Geometry check sheet. Reference: the model listing, model coordinates, mm. A direction names the side the tool comes from. Give positions to 0.01 mm unless a question says otherwise; leave off trailing zeros. Write each loop counter-clockwise with the first axis right and the second up, starting at its lowest first coordinate (ties: lowest second). Pieces come first, ordered by that corner, then holes. Notation, with made-up numbers: (56, 20) - (60, 20) arc R20 ccw to (60, 55) - close; hole circle Ø5 at (64, 39.5). An arc over 180 degrees is marked (long way). One line per question, with ' | ' between items. Start each with the question number.
Q1. Release check for a two-part mould opening along X. For faces 5 (the face through (-2.1, -12.4, 0)), 6 (the face through (0, -7, -14)), 7 (the face through (-8.767, -16.856, 2.902)) record: +X half, -X half, draft (parallel to the pull), parting line (faces both ways), or undercut.
Q2. Section check C-C on z = -1.25. Record the boundary of the cut face in (x, y).
Q3. Thickness scan on L1, parallel to Y at x = 0, z = -11.65; L2, parallel to X at y = -11, z = 6.5; L3, parallel to Y at x = -11, z = -0.75. Record the ranges inside material, lowest first. Write a range as [from, to].
Q4. Set-up check for faces 1 (the face through (-5.72, -11, 0.74)), 2 (the face through (-10.7, 10.4, 2.9)), 3 (the face through (1.5, 9, -13.5)), 4 (the face through (-5.602, 0.9, -13.5)): record each of +Z, -Z, +X, -X, +Y, -Y from which the full face is reachable in a straight line by a thin tool's end or side.
Q5. Gauge pin test, flat ends, axial feed: P1, Ø8.5, axis at x = 5, y = 4.5, coming from the +Z side; P2, Ø1, axis at x = 7, z = -2.5, coming from the +Y side; P3, Ø1.1, axis at y = 1.5, z = -13.5, coming from the -X side. Record the tip position at first contact, or that the pin passes through.
Q6. Section check D-D on x = 15. Record the boundary of the cut face in (y, z).
```python
from build123d import *

# Parameters (mm, degrees)
F2_R     = 1.1
F3_DEPTH = 14
F5_DEPTH = 1


with BuildPart() as f1:
    # F0 (on Front) → F1 (revolve)
    with BuildSketch(Plane.XZ):
        with BuildLine():
            Line((-14, 0), (-14, 9.5))
            ThreePointArc((-14, 9.5), (-14.146447, 9.853553), (-14.5, 10))
            Line((-14.5, 10), (-19, 10))
            Line((-19, 10), (-19, -4))
            Line((-19, -4), (-11, -4))
            Line((-11, -4), (-11, -14))
            Line((-11, -14), (-4, -14))
            Line((-4, -14), (-4, -8.1))
            Line((-4, -8.1), (-9.6, -2.5))
            Line((-9.6, -2.5), (-9.6, 1.5))
            ThreePointArc((-9.6, 1.5), (-9.746447, 1.853553), (-10.1, 2))
            Line((-10.1, 2), (-11.9, 2))
            ThreePointArc((-11.9, 2), (-12.253553, 1.853553), (-12.4, 1.5))
            Line((-12.4, 1.5), (-12.4, 0))
            Line((-12.4, 0), (-14, 0))
        make_face()
    revolve(axis=Axis((0, 0, -7), (0, 0, -1)))

    # F2 (on face) → F3 (cut, through all)
    with BuildSketch(Plane(origin=(0, 0, -4), x_dir=(1, 0, 0), z_dir=(0, 0, -1))):
        with Locations((11.313708, 11.313708)):
            Circle(F2_R)
        with Locations((-11.313708, -11.313708)):
            Circle(F2_R)
        with Locations((11.313708, -11.313708)):
            Circle(F2_R)
        with Locations((-11.313708, 11.313708)):
            Circle(F2_R)
    extrude(amount=-F3_DEPTH, mode=Mode.SUBTRACT)

    # F4 (on face) → F5 (cut)
    with BuildSketch(Plane(origin=(0, 0, -14), x_dir=(1, 0, 0), z_dir=(0, 0, -1))):
        with BuildLine():
            Line((4.332, 5.01), (-4.332, 5.01))
            ThreePointArc((-4.332, 5.01), (-5.230026, 4.638026), (-5.602, 3.74))
            Line((-5.602, 3.74), (-5.602, -5.72))
            ThreePointArc((-5.602, -5.72), (-5.230026, -6.618026), (-4.332, -6.99))
            Line((-4.332, -6.99), (-1.5, -6.99))
            Line((-1.5, -6.99), (-1.5, -11.99))
            ThreePointArc((-1.5, -11.99), (0, -13.49), (1.5, -11.99))
            Line((1.5, -11.99), (1.5, -6.99))
            Line((1.5, -6.99), (4.332, -6.99))
            ThreePointArc((4.332, -6.99), (5.230026, -6.618026), (5.602, -5.72))
            Line((5.602, -5.72), (5.602, 3.74))
            ThreePointArc((5.602, 3.74), (5.230026, 4.638026), (4.332, 5.01))
        make_face()
    extrude(amount=-F5_DEPTH, mode=Mode.SUBTRACT)


solid = f1.part
```
Working result:
1) face 5: undercut | face 6: draft | face 7: parting line
2) outline: circle Ø38 at (0, 0); hole circle Ø2.2 at (-11.31, -11.31); hole circle Ø2.2 at (-11.31, 11.31); hole circle Ø19.2 at (0, 0); hole circle Ø2.2 at (11.31, -11.31); hole circle Ø2.2 at (11.31, 11.31)
3) L1: y = [-11, -4], [4, 11] | L2: x = [-15.49, -12.37], [-10.26, -8.66], [8.66, 10.26], [12.37, 15.49] | L3: y = [-15.49, -12.37], [-10.26, 10.26], [12.37, 15.49]
4) face 1: +Z | face 2: +Z, -Z | face 3: -Z, +Y | face 4: -Z
5) P1: stops at z = 2 | P2: stops at y = 17.85 | P3: stops at x = -10.96
6) outline: (-11.66, -4) - (11.66, -4) - (11.66, 10) - (-11.66, 10) - close
